Print and shaded views of the part. All mm, measured from the part's lowest x, y and z. Coordinates: 2 decimals unless noted, no trailing zeros. Order: outer loops, then holes, each group sorted by start corner. A loop starts at its lowest first (then second) coordinate and runs counter-clockwise, first axis right, second up.
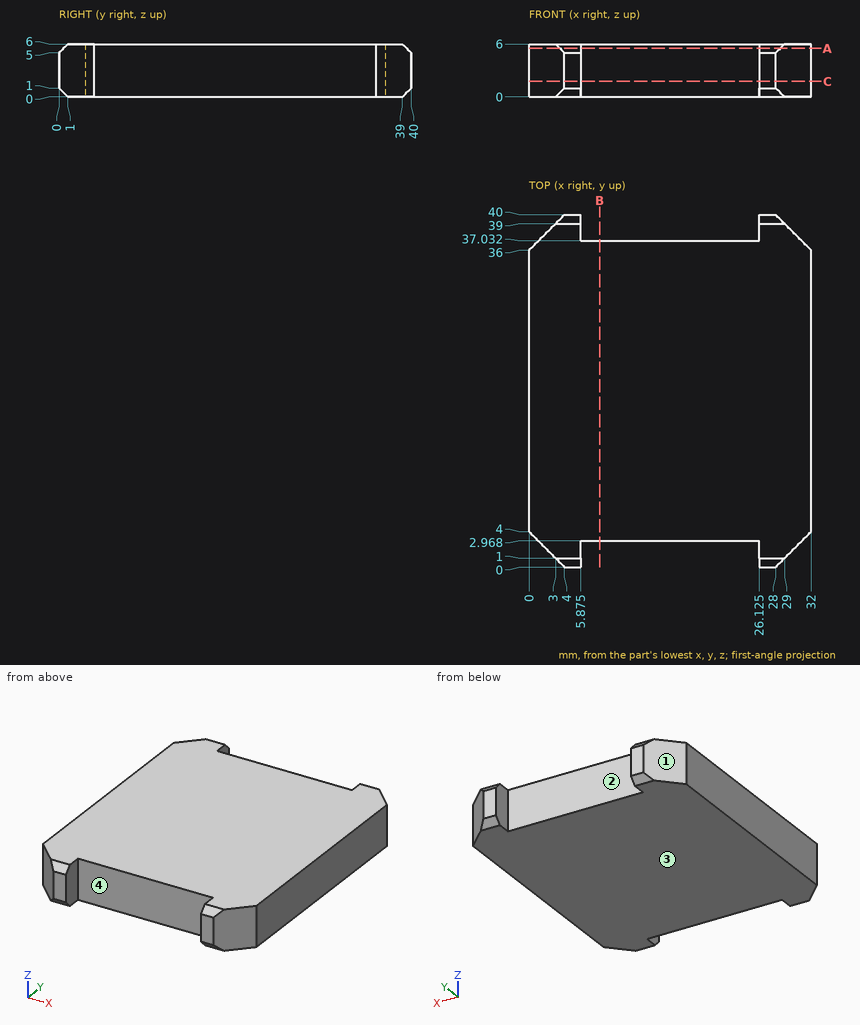
Q1. Mould opens along X. For the marked faces 1, 2, 3 and 4 say: pulls with the +X half, pulls with the -X half, needs draft (parallel to the pull), parting line crosses it, or undercut.
Established:
face 1: pulls with the -X half
face 2: undercut
face 3: needs draft
face 4: undercut
Q2. Cut at B-B, the plane x = 8. List the corners of the cut face in (y, z).
Established:
outline: (2.97, 0) - (37.03, 0) - (37.03, 6) - (2.97, 6) - close
Q3. Probe line 1 (Y direction, x = 17, z = 2); line 2 (X direction, y = 2.5, z = 3.75) (1 decimal); line 3 (Y direction, x = 5, z = 0.75). List the from-to ranges inside material, lowest first.
Established:
line 1: y = 2.97 to 37.03
line 2: x = 1.5 to 5.9, 26.1 to 30.5
line 3: y = 0.25 to 39.75
Q4. Drop flat-ended pins along their axis: P1, Ø1.5, axis at y = 2, z = 1.5, coming from the +X side; P2, Ø3.5, axis at y = 38, z = 4.5, coming from the -X side; P3, Ø3.5, axis at y = 38.5, z = 3.5, coming from the +X side. Give the stop position or say it passes through.
Established:
P1: stops at x = 30.75
P2: stops at x = 0.25
P3: stops at x = 31.25
Q5. Cut at A-A, the plane z = 5.5. List the corners of the cut face in (x, y) (1 decimal).
Established:
outline: (0, 4) - (3.5, 0.5) - (5.9, 0.5) - (5.9, 3) - (26.1, 3) - (26.1, 0.5) - (28.5, 0.5) - (32, 4) - (32, 36) - (28.5, 39.5) - (26.1, 39.5) - (26.1, 37) - (5.9, 37) - (5.9, 39.5) - (3.5, 39.5) - (0, 36) - close
Q6. Cut at C-C, the plane z = 1.75. List the corners of the cut face in (x, y) (1 decimal).
Established:
outline: (0, 4) - (4, 0) - (5.9, 0) - (5.9, 3) - (26.1, 3) - (26.1, 0) - (28, 0) - (32, 4) - (32, 36) - (28, 40) - (26.1, 40) - (26.1, 37) - (5.9, 37) - (5.9, 40) - (4, 40) - (0, 36) - close
